Verification items for the finished model (mm, model axes). A direction names the side the tool comes from. Give positions to 0.01 mm unless a question says otherwise; leave off trailing zeros. Loops run counter-clockwise (first coordinate to the right, second up) from the corner with the lowest first, then second, coordinate; pieces in that order, holes last. Notation, with made-up numbers: M 53,47.25 L 104,47.25 A22 cw 104,85.25 Z; hole C 1,72.5 d8. An arc over 180 degrees is marked long. Answer in a Markdown table with one row per item.
```python
from build123d import *

# Parameters (mm, degrees)
SWEEP2_PROFILE_R = 15
SWEEP3_PROFILE_R = 6
SWEEP4_PROFILE_R = 5
SWEEP5_PROFILE_R = 5


with BuildPart() as part:
    # Sweep2: sweep along a path in Sketch1
    with BuildLine(Plane.XY) as sweep2_path:
        Line((0, 20), (0, -20))
    # Sweep2 profile (on start of the path) → Sweep2 (sweep)
    with BuildSketch(Plane(origin=(0, 20, 0), x_dir=(-1, 0, 0), z_dir=(0, -1, 0))):
        Circle(SWEEP2_PROFILE_R)
    sweep(path=sweep2_path.line)

    # Sweep3: sweep along a path in Sketch30
    with BuildLine(Plane.XY) as sweep3_path:
        Line((0, 0), (88, 0))
    # Sweep3 profile (on start of the path) → Sweep3 (sweep)
    with BuildSketch(Plane(origin=(0, 0, 0), x_dir=(0, 0, 1), z_dir=(1, 0, 0))):
        Circle(SWEEP3_PROFILE_R)
    sweep(path=sweep3_path.line)

    # Sweep4: sweep along a path in Sketch39
    with BuildLine(Plane.XY) as sweep4_path:
        Line((0, -20), (0, -74))
    # Sweep4 profile (on start of the path) → Sweep4 (sweep)
    with BuildSketch(Plane(origin=(0, -20, 0), x_dir=(0, 0, -1), z_dir=(0, -1, 0))):
        Circle(SWEEP4_PROFILE_R)
    sweep(path=sweep4_path.line)

    # Sweep5: sweep along a path in Sketch45
    with BuildLine(Plane.XY) as sweep5_path:
        Line((0, 20), (0, 74))
    # Sweep5 profile (on start of the path) → Sweep5 (sweep)
    with BuildSketch(Plane.ZX.offset(20)):
        Circle(SWEEP5_PROFILE_R)
    sweep(path=sweep5_path.line)


solid = part.part
```
Item 1: Sectioned sample at C-C (y = 0). Record the cut outline in (x, z).
Reported:
| item | result |
|---|---|
| outline | M 13.75,-6 L 88,-6 L 88,6 L 13.75,6 A15 ccw long Z |
Item 2: Go/stop test with flat-tipped pins: pin 1 (5 mm diameter, centred on x = 27.5, z = 7.5, fed in from +Y); pin 2 (2 mm diameter, centred on y = 44.5, z = -2, fed in from +X); pin 3 (5 mm diameter, centred on x = 39, y = 5.5, fed in from -Z); pin 4 (15 mm diameter, centred on x = 2, z = -6, fed in from +Y). Record where each tip stops, or that it passes through.
Reported:
| item | result |
|---|---|
| pin 1 | stops at y = 3.32 |
| pin 2 | stops at x = 4.9 |
| pin 3 | stops at z = -5.2 |
| pin 4 | stops at y = 74 |
Item 3: Sectioned sample at D-D (x = 33.5). Record the cut outline in (y, z), and give its area (3 significant figures).
Reported:
| item | result |
|---|---|
| outline | C 0,0 d12 |
| area | 113 mm^2 |
Item 4: Scan lines: L1, parallel to Y at x = -10, z = 10; L2, parallel to X at y = -52, z = 0; L3, parallel to X at y = -11, z = 5. Record each from-to range of solid material in increasing order. Write a range as [from, to].
Reported:
| item | result |
|---|---|
| L1 | y = [-20, 20] |
| L2 | x = [-5, 5] |
| L3 | x = [-14.14, 14.14] |
Item 5: Tool access check on faces 1 (the cylindrical face through (-4.88, 47.38, -1.08)), 2 (the cylindrical face through (51, 0, -6)), 3 (the flat face through (4, -20, 4)). Record the directions out of +Z, -Z, +X, -X, +Y, -Y that give a thin tool (end or side, any length) a straight path to the whole face; none if there is none.
Reported:
| item | result |
|---|---|
| face 1 | +Y |
| face 2 | +X |
| face 3 | -Y |
Item 6: Sectioned sample at A-A (x = 0). Record the cut outline in (y, z).
Reported:
| item | result |
|---|---|
| outline | M -74,-5 L -20,-5 L -20,-15 L 20,-15 L 20,-5 L 74,-5 L 74,5 L 20,5 L 20,15 L -20,15 L -20,5 L -74,5 Z |
Item 7: Sectioned sample at B-B (z = 0). Record the cut outline in (x, y).
Reported:
| item | result |
|---|---|
| outline | M -15,-20 L -5,-20 L -5,-74 L 5,-74 L 5,-20 L 15,-20 L 15,-6 L 88,-6 L 88,6 L 15,6 L 15,20 L 5,20 L 5,74 L -5,74 L -5,20 L -15,20 Z |
